Verification items for the finished model (mm, model axes). A direction names the side the tool comes from. Round coordinates to 2 decimals unless told otherwise and drop trailing zeros. Loops run counter-clockwise (first coordinate to the right, second up) from the corner with the lowest first, then second, coordinate; pieces in that order, holes last. Notation, with made-up numbers: M 4.5,74.5 L 32.5,74.5 A24 cw 32.5,98.5 Z; hole C -15,89.25 d8. An arc over 180 degrees is marked long. One line per item, written item: value.
from build123d import *

# Parameters (mm, degrees)
F0_W     = 25
F0_H     = 5.803798
F1_DEPTH = 1.35
F2_DEPTH = 0.85


with BuildPart() as f1:
    # F0 (on Front) → F1 (new body)
    with BuildSketch(Plane.XZ):
        Rectangle(F0_W, F0_H)
    extrude(amount=F1_DEPTH)

    # F0 (on Front) → F2 (join)
    with BuildSketch(Plane.XZ):
        with BuildLine():
            Line((25, 1.55), (25, 3.5))
            Line((25, 3.5), (-25, 3.5))
            Line((-25, 3.5), (-25, 1.55))
            Line((-25, 1.55), (-23, 1.55))
            ThreePointArc((-23, 1.55), (-21.45, 0), (-23, -1.55))
            Line((-23, -1.55), (-25, -1.55))
            Line((-25, -1.55), (-25, -3.5))
            Line((-25, -3.5), (25, -3.5))
            Line((25, -3.5), (25, -1.55))
            Line((25, -1.55), (23, -1.55))
            ThreePointArc((23, -1.55), (21.45, 0), (23, 1.55))
            Line((23, 1.55), (25, 1.55))
        make_face()
        Rectangle(F0_W, F0_H, mode=Mode.SUBTRACT)
    extrude(amount=F2_DEPTH)


solid = f1.part
(1) Mould release check, pull along Z, two halves, no side actions. Record for faces 1 (the face through (-0.3, -0.4, -3.5)), 2 (the face through (-24, -0.4, -1.55)), 3 (the face through (0, 0, 0)): +Z half, -Z half, draft (parallel to the pull), parting line (faces both ways), or undercut.
Completed:
face 1: -Z half
face 2: undercut
face 3: draft
(2) Sectioned sample at B-B on z = 2. Enter the section's corners in (x, y).
Completed:
outline: M -25,-0.85 L -12.5,-0.85 L -12.5,-1.35 L 12.5,-1.35 L 12.5,-0.85 L 25,-0.85 L 25,0 L -25,0 Z
(3) Tool access check on faces 4 (the face through (-25, -0.4, -2.5)), 5 (the face through (-24, -0.4, 1.55)), 6 (the face through (24, -0.4, 1.55)). Record the directions out of +Z, -Z, +X, -X, +Y, -Y that give a thin tool (end or side, any length) a straight path to the whole face; none if there is none.
Completed:
face 4: +Z, -Z, -X, +Y, -Y
face 5: -X, +Y, -Y
face 6: +X, +Y, -Y
(4) Sectioned sample at A-A on x = 6.5. Enter the section's corners in (y, z), and give its area (3 significant figures).
Completed:
outline: M -1.35,-2.9 L -0.85,-2.9 L -0.85,-3.5 L 0,-3.5 L 0,3.5 L -0.85,3.5 L -0.85,2.9 L -1.35,2.9 Z
area: 8.85 mm^2
(5) Sectioned sample at C-C on y = -0.6. Enter the section's corners in (x, z).
Completed:
outline: M -25,-3.5 L 25,-3.5 L 25,-1.55 L 23,-1.55 A1.55 cw 23,1.55 L 25,1.55 L 25,3.5 L -25,3.5 L -25,1.55 L -23,1.55 A1.55 cw -23,-1.55 L -25,-1.55 Z
(6) Thickness scan on L1, parallel to Z at x = -3, y = -1.1; L2, parallel to X at y = -1.05, z = -1.5; L3, parallel to Y at x = -16, z = -1.75. Record the ranges inside material, lowest first. Write a range as from..to.
Completed:
L1: z = -2.9..2.9
L2: x = -12.5..12.5
L3: y = -0.85..0
(7) Depth check by flat-ended pin: pin 1 Ø0.6 at (y, z) = (-1, 0) entering from -X; pin 2 Ø1 at (x, z) = (15, 2) entering from -Y. Enter the tip coordinate at first touch or a pass-through.
Completed:
pin 1: stops at x = -21.47
pin 2: stops at y = -0.85
